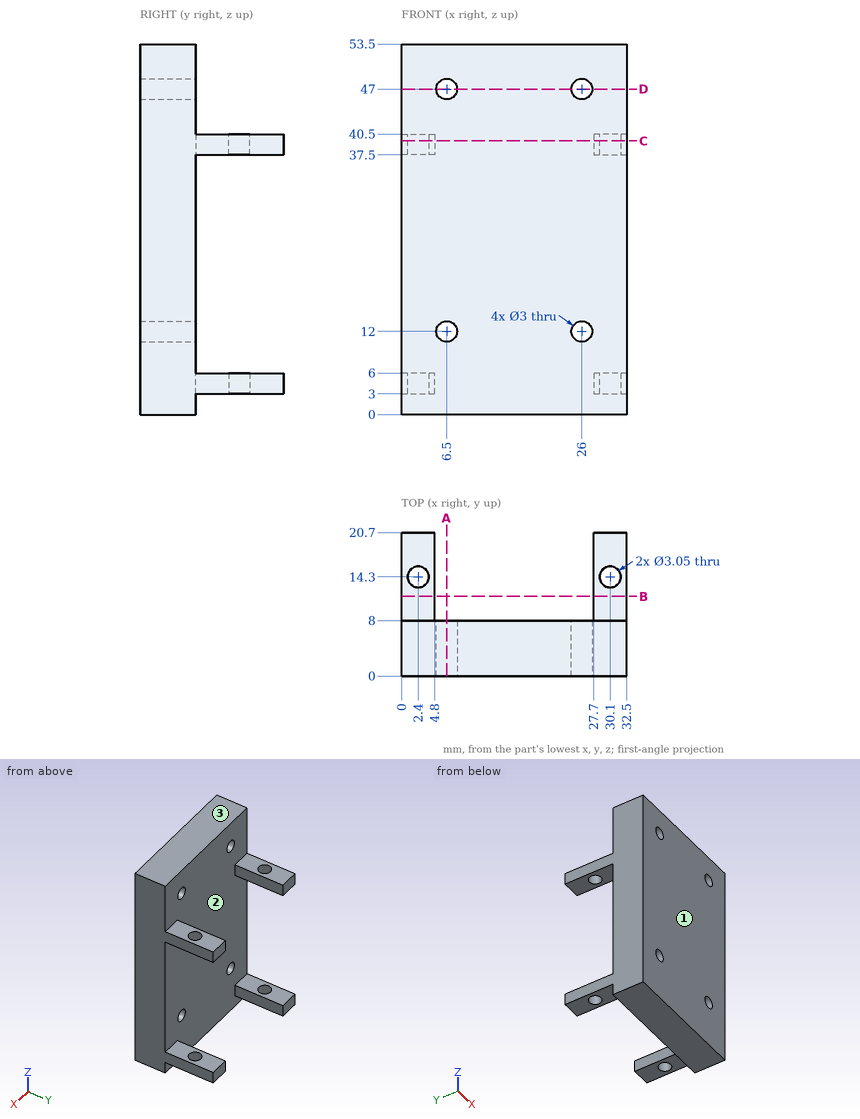
Design review of the part shown in the three views and the two pictorial views. Dimensions are in mm from the part's minimum x, y and z. Give positions to 0.01 mm unless a question says otherwise; leave off trailing zeros. Loops run counter-clockwise (first coordinate to the right, second up) from the corner with the lowest first, then second, coordinate; pieces in that order, holes last. Notation, with made-up numbers: (48.5, -27) -> (91.5, -27) arc R23 ccw to (91.5, -19) -> close; hole circle Ø11 at (55, 83.25). An arc over 180 degrees is marked (long way). Put each result on its own line as item: value. Start each with the question number.
1. Clearance check with flat-ended pins moving along their axes: P1, Ø12, axis at x = 19, z = 45.5, coming from the +Y side; P2, Ø5.5, axis at x = 1.5, y = 14.5, coming from the +Z side; P3, Ø5, axis at x = 30.1, y = 14.3, coming from the -Z side. State where each tip first meets the part, or that it passes through.
2. We need section A-A on x = 6.5. State the section outline as (y, z) points, then the cut area to 3 significant figures.
3. Mouldability with a two-part tool opening along Z and no side actions: class the marked faces 1, 2 and 3 as released by +Z, released by -Z, zero draft, split by the parting line, or undercut.
4. Wall thickness on probe 1 along Z at (x, y) = (6.5, 4.5); probe 2 along X at (y, z) = (5, 12); probe 3 along Y at (x, z) = (2.4, 5.05) (3 decimals): over which ranges is each line inside the solid? List them lowest first.
5. We need section D-D on z = 47. State the section outline as (x, y) points, then the cut area to 3 significant figures.
6. We need section B-B on y = 11.5. State the section outline as (x, z) points.
7. We need section C-C on z = 39.5. State the section outline as (x, y) points (3 decimals), then the cut area to 3 significant figures.
Determined:
1. P1: y = 8
1. P2: z = 40.5
1. P3: z = 3
2. outline: (0, 0) -> (8, 0) -> (8, 10.5) -> (0, 10.5) -> close; (0, 13.5) -> (8, 13.5) -> (8, 45.5) -> (0, 45.5) -> close; (0, 48.5) -> (8, 48.5) -> (8, 53.5) -> (0, 53.5) -> close
2. area: 380 mm^2
3. face 1: zero draft
3. face 2: undercut
3. face 3: released by +Z
4. probe 1: 0 to 10.5, 13.5 to 45.5, 48.5 to 53.5
4. probe 2: 0 to 5, 8 to 24.5, 27.5 to 32.5
4. probe 3: 0 to 12.775, 15.825 to 20.7
5. outline: (0, 0) -> (5, 0) -> (5, 8) -> (0, 8) -> close; (8, 0) -> (24.5, 0) -> (24.5, 8) -> (8, 8) -> close; (27.5, 0) -> (32.5, 0) -> (32.5, 8) -> (27.5, 8) -> close
5. area: 212 mm^2
6. outline: (0, 3) -> (4.8, 3) -> (4.8, 6) -> (0, 6) -> close; (0, 37.5) -> (4.8, 37.5) -> (4.8, 40.5) -> (0, 40.5) -> close; (27.7, 3) -> (32.5, 3) -> (32.5, 6) -> (27.7, 6) -> close; (27.7, 37.5) -> (32.5, 37.5) -> (32.5, 40.5) -> (27.7, 40.5) -> close
7. outline: (0, 0) -> (32.5, 0) -> (32.5, 20.7) -> (27.7, 20.7) -> (27.7, 8) -> (4.8, 8) -> (4.8, 20.7) -> (0, 20.7) -> close; hole circle Ø3.05 at (2.4, 14.3); hole circle Ø3.05 at (30.1, 14.3)
7. area: 367 mm^2
